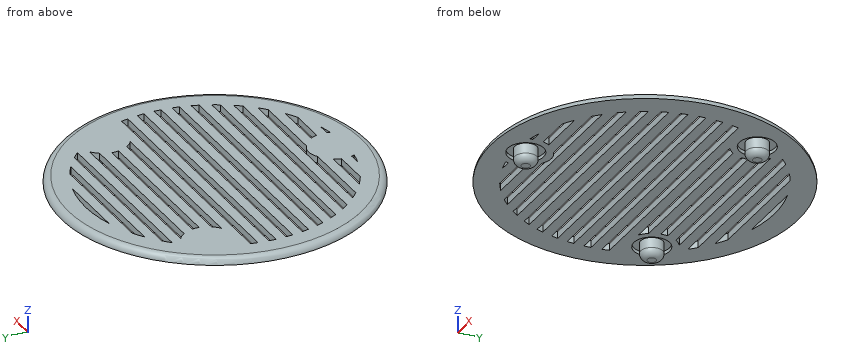
from build123d import *

# Parameters (mm, degrees)
F0_R     = 45
F1_DEPTH = 2
F2_R     = 5.25
F3_DEPTH = 1
F4_R     = 3.25
F5_DEPTH = 5
F6_R     = 2
F7_R     = 1.99999
F9_DEPTH = 25


# Not quite as in the source:
# - a fillet or chamfer is up to 0.001 mm smaller than in the source, because OpenCascade refuses the exact size


with BuildPart() as f1:
    # F0 (on Top) → F1 (new body)
    with BuildSketch(Plane.XY):
        Circle(F0_R)
    extrude(amount=F1_DEPTH)

    # F2 (on face) → F3 (cut)
    with BuildSketch(Plane(origin=(0, 0, 0), x_dir=(1, 0, 0), z_dir=(0, 0, -1))):
        with Locations((0, 35)):
            Circle(F2_R)
        with Locations((-30.3108891325, -17.5)):
            Circle(F2_R)
        with Locations((30.3108891325, -17.5)):
            Circle(F2_R)
    extrude(amount=-F3_DEPTH, mode=Mode.SUBTRACT)

    # F4 (on face) → F5 (join)
    with BuildSketch(Plane(origin=(0, 0, 1), x_dir=(1, 0, 0), z_dir=(0, 0, -1))):
        with Locations((0, 35)):
            Circle(F4_R)
        with Locations((30.3108891325, -17.5)):
            Circle(F4_R)
        with Locations((-30.3108891325, -17.5)):
            Circle(F4_R)
    extrude(amount=F5_DEPTH)

    # F6
    f6_edges = [f1.edges().sort_by_distance(p)[0] for p in [
        (-33.560889, 17.5, -4),
        (-3.25, -35, -4),
        (27.060889, 17.5, -4),
    ]]
    fillet(f6_edges, radius=F6_R)

    # F7 (radius 2 in the source; OpenCascade refuses exactly that, so slightly less here)
    f7_edges = [f1.edges().sort_by_distance(p)[0] for p in [
        (-45, 0, 2),
    ]]
    fillet(f7_edges, radius=F7_R)

    # F8 (on face) → F9 (cut)
    with BuildSketch(Plane.XY.offset(2)):
        with BuildLine():
            Line((17.9373911147, 33.5), (-17.9373911147, 33.5))
            ThreePointArc((-17.9373911147, 33.5), (-19.6214001606, 32.5422902657), (-21.2544113068, 31.5))
            Line((-21.2544113068, 31.5), (21.2544113068, 31.5))
            ThreePointArc((21.2544113068, 31.5), (19.6214001606, 32.5422902657), (17.9373911147, 33.5))
        make_face()
        with BuildLine():
            Line((-7.0931304796, -36.5), (-10.5711872559, -36.5))
            ThreePointArc((-10.5711872559, -36.5), (-8.7211541333, -36.9856927823), (-6.8490250847, -37.3776785714))
            ThreePointArc((-6.8490250847, -37.3776785714), (-6.9848769039, -36.9426771829), (-7.0931304796, -36.5))
        make_face()
        with BuildLine():
            ThreePointArc((-21.2544113068, -31.5), (-19.6214001606, -32.5422902657), (-17.9373911147, -33.5))
            Line((-17.9373911147, -33.5), (-7.0931304796, -33.5))
            ThreePointArc((-7.0931304796, -33.5), (-6.7951561077, -32.4724807673), (-6.3492125496, -31.5))
            Line((-6.3492125496, -31.5), (-21.2544113068, -31.5))
        make_face()
        with BuildLine():
            ThreePointArc((-27.2350876628, -26.5), (-26.2039506035, -27.5200467436), (-25.1346374551, -28.5))
            Line((-25.1346374551, -28.5), (-3.2113081447, -28.5))
            ThreePointArc((-3.2113081447, -28.5), (0, -27.5), (3.2113081447, -28.5))
            Line((3.2113081447, -28.5), (25.1346374551, -28.5))
            ThreePointArc((25.1346374551, -28.5), (26.2039506035, -27.5200467436), (27.2350876628, -26.5))
            Line((27.2350876628, -26.5), (-27.2350876628, -26.5))
        make_face()
        with BuildLine():
            ThreePointArc((-31.3328900678, -21.5), (-30.6138735789, -22.5120133372), (-29.8621834433, -23.5))
            Line((-29.8621834433, -23.5), (29.8621834433, -23.5))
            ThreePointArc((29.8621834433, -23.5), (30.6138735789, -22.5120133372), (31.3328900678, -21.5))
            Line((31.3328900678, -21.5), (-31.3328900678, -21.5))
        make_face()
        with BuildLine():
            ThreePointArc((-34.2308340535, -16.5), (-33.7265552305, -17.5076975151), (-33.1926196616, -18.5))
            Line((-33.1926196616, -18.5), (33.1926196616, -18.5))
            ThreePointArc((33.1926196616, -18.5), (33.7265552305, -17.5076975151), (34.2308340535, -16.5))
            Line((34.2308340535, -16.5), (-34.2308340535, -16.5))
        make_face()
        with BuildLine():
            ThreePointArc((-36.2180894029, -11.5), (-35.8835416114, -12.5048567133), (-35.5211204778, -13.5))
            Line((-35.5211204778, -13.5), (35.5211204778, -13.5))
            ThreePointArc((35.5211204778, -13.5), (35.8835416114, -12.5048567133), (36.2180894029, -11.5))
            Line((36.2180894029, -11.5), (-36.2180894029, -11.5))
        make_face()
        with BuildLine():
            ThreePointArc((-37.439951923, -6.5), (-37.2519722478, -7.5027037562), (-37.0371435184, -8.5))
            Line((-37.0371435184, -8.5), (37.0371435184, -8.5))
            ThreePointArc((37.0371435184, -8.5), (37.2519722478, -7.5027037562), (37.439951923, -6.5))
            Line((37.439951923, -6.5), (-37.439951923, -6.5))
        make_face()
        with BuildLine():
            ThreePointArc((-37.9703831953, -1.5), (-37.9176166167, -2.5008698704), (-37.838472485, -3.5))
            Line((-37.838472485, -3.5), (37.838472485, -3.5))
            ThreePointArc((37.838472485, -3.5), (37.9176166167, -2.5008698704), (37.9703831953, -1.5))
            Line((37.9703831953, -1.5), (-37.9703831953, -1.5))
        make_face()
        with BuildLine():
            ThreePointArc((-37.838472485, 3.5), (-37.9176166167, 2.5008698704), (-37.9703831953, 1.5))
            Line((-37.9703831953, 1.5), (37.9703831953, 1.5))
            ThreePointArc((37.9703831953, 1.5), (37.9176166167, 2.5008698704), (37.838472485, 3.5))
            Line((37.838472485, 3.5), (-37.838472485, 3.5))
        make_face()
        with BuildLine():
            ThreePointArc((-37.0371435184, 8.5), (-37.2519722478, 7.5027037562), (-37.439951923, 6.5))
            Line((-37.439951923, 6.5), (37.439951923, 6.5))
            ThreePointArc((37.439951923, 6.5), (37.2519722478, 7.5027037562), (37.0371435184, 8.5))
            Line((37.0371435184, 8.5), (-37.0371435184, 8.5))
        make_face()
        with BuildLine():
            Line((24.2641958212, 13.5), (-24.2641958212, 13.5))
            ThreePointArc((-24.2641958212, 13.5), (-25.1547879454, 12.403224495), (-26.2411839834, 11.5))
            Line((-26.2411839834, 11.5), (26.2411839834, 11.5))
            ThreePointArc((26.2411839834, 11.5), (25.1547879454, 12.403224495), (24.2641958212, 13.5))
        make_face()
        with BuildLine():
            ThreePointArc((-23.1301858243, 18.5), (-23.0608891325, 17.5), (-23.1301858243, 16.5))
            Line((-23.1301858243, 16.5), (23.1301858243, 16.5))
            ThreePointArc((23.1301858243, 16.5), (23.0608891325, 17.5), (23.1301858243, 18.5))
            Line((23.1301858243, 18.5), (-23.1301858243, 18.5))
        make_face()
        with BuildLine():
            ThreePointArc((-26.2411839834, 23.5), (-25.1547879454, 22.596775505), (-24.2641958212, 21.5))
            Line((-24.2641958212, 21.5), (24.2641958212, 21.5))
            ThreePointArc((24.2641958212, 21.5), (25.1547879454, 22.596775505), (26.2411839834, 23.5))
            Line((26.2411839834, 23.5), (-26.2411839834, 23.5))
        make_face()
        with BuildLine():
            ThreePointArc((-25.1346374551, 28.5), (-26.2039506035, 27.5200467436), (-27.2350876628, 26.5))
            Line((-27.2350876628, 26.5), (27.2350876628, 26.5))
            ThreePointArc((27.2350876628, 26.5), (26.2039506035, 27.5200467436), (25.1346374551, 28.5))
            Line((25.1346374551, 28.5), (-25.1346374551, 28.5))
        make_face()
        with BuildLine():
            ThreePointArc((10.5711872559, 36.5), (0, 38), (-10.5711872559, 36.5))
            Line((-10.5711872559, 36.5), (10.5711872559, 36.5))
        make_face()
        with BuildLine():
            Line((7.0931304796, -33.5), (17.9373911147, -33.5))
            ThreePointArc((17.9373911147, -33.5), (19.6214001606, -32.5422902657), (21.2544113068, -31.5))
            Line((21.2544113068, -31.5), (6.3492125496, -31.5))
            ThreePointArc((6.3492125496, -31.5), (6.7951561077, -32.4724807673), (7.0931304796, -33.5))
        make_face()
        with BuildLine():
            Line((10.5711872559, -36.5), (7.0931304796, -36.5))
            ThreePointArc((7.0931304796, -36.5), (6.9848769039, -36.9426771829), (6.8490250847, -37.3776785714))
            ThreePointArc((6.8490250847, -37.3776785714), (8.7211541333, -36.9856927823), (10.5711872559, -36.5))
        make_face()
    extrude(amount=-F9_DEPTH, mode=Mode.SUBTRACT)


solid = f1.part
The listing builds one solid part. Answer for the finished solid, in the listing's coordinates (mm). Coordinates: 2 decimals unless noted, no trailing zeros. Answer in a Markdown table with one row per item. Add a question column.
1. Consider line 1 (X direction, y = -35, z = 0.25); line 2 (X direction, y = -35, z = 0.75); line 3 (X direction, y = 17.5, z = 0.35). Determine where each line is inside the solid, lowest interval first. Write a range as [from, to].
2. The part is cut by section B-B, the plane z = -3.1. Count the separate pieces of the cut face and the enclosed holes in it, then the cut area to 3 significant figures.
3. Flat-ended cylindrical pins translate along their axes: P1, Ø0.6, axis at x = 2, z = 1, coming from the -Y side; P2, Ø1, axis at x = -17.5, z = 1.5, coming from the -Y side; P3, Ø0.6, axis at x = 17.5, z = 0.5, coming from the +Y side. Find the tip coordinate at first contact, or state that the pin passes through.
Answer below:
| question | item | result |
|---|---|---|
| 1 | line 1 | [-28.26, -5.25], [-3.25, 3.25], [5.25, 28.26] |
| 1 | line 2 | [-28.05, -5.25], [-3.25, 3.25], [5.25, 28.05] |
| 1 | line 3 | [-41.42, -35.56], [-33.56, -27.06], [-25.06, -23.06], [23.06, 25.06], [27.06, 33.56], [35.56, 41.42] |
| 2 | separate pieces | 3 |
| 2 | enclosed holes | 0 |
| 2 | area | 80.4 mm2 |
| 3 | P1 | y = -44.83 |
| 3 | P2 | y = -41.23 |
| 3 | P3 | y = 41.53 |
